Design review of the part built by this model. Coordinates are the model's own, in mm. Face numbers are marked on the shaded views. A direction names the side the tool comes from. Coordinates: 2 decimals unless noted, no trailing zeros. Loops run counter-clockwise (first coordinate to the right, second up) from the corner with the lowest first, then second, coordinate; pieces in that order, holes last. Notation, with made-up numbers: (-25, 4.25) -> (3, 4.25) arc R23 cw to (3, 20.25) -> close; hole circle Ø7 at (85, -11.5). An arc over 180 degrees is marked (long way). One line per item, written item: value. Start each with the question number.
1. Add section A-A on z = -70.5. Write out the cut boundary in (x, y).
2. Draft analysis for pull direction Y (two halves, no side actions). For the marked faces 1, 2, 3 and 4, state which applies: pulls with the +Y half, pulls with the -Y half, needs draft (parallel to the pull), parting line crosses it, or undercut.
3. Insertion check: pin 1 (6 mm diameter, centred on x = -157, z = -24, fed in from -Y); pin 2 (4 mm diameter, centred on y = -91.5, z = 2, fed in from +X); pin 3 (8 mm diameter, centred on x = -125, y = 0, fed in from +Z). Each pin has a flat end and moves straight along its axis. Give the tip position at first contact, or say it passes through.
4. Machinability: for the marked faces 5, 6, 7, 8 and 9, which of the approach directions +Z, -Z, +X, -X, +Y, -Y give a long, thin tool a straight path to every point of the face, cutting with its end or side? Answer none if there is none.
5. Add section B-B on z = 41. Write out the cut boundary in (x, y).
6. For probe 1 along Z at (x, y) = (-264.5, 45); probe 2 along X at (y, z) = (-70, -5.5); probe 3 along Y at (x, z) = (-195.5, 32), list the stretches that pass through material, from the lowest coordinate up.
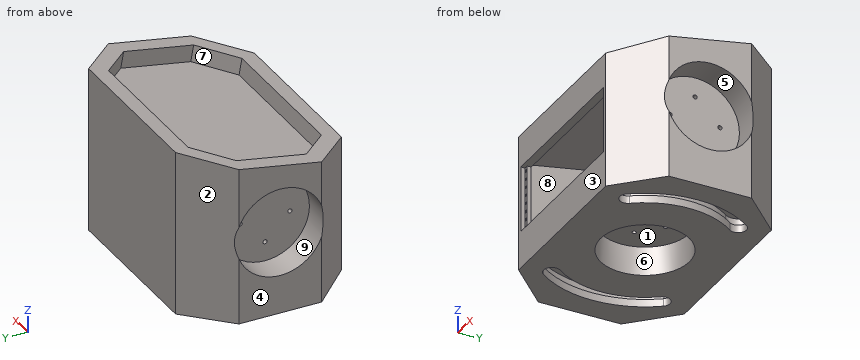
```python
from build123d import *

# Parameters (mm, degrees)
SKETCH1_W           = 200
SKETCH1_H           = 200
BOSS_EXTRUDE1_DEPTH = 150
SKETCH2_R           = 53.5
CUT_EXTRUDE1_DEPTH  = 35
CUT_EXTRUDE3_DEPTH  = 332.662479036
CHAMFER2_SIZE       = 50
CUT_EXTRUDE5_DEPTH  = 20
CUT_EXTRUDE6_DEPTH  = 20
BOSS_EXTRUDE3_DEPTH = 9.2
SKETCH11_R          = 53.5
CUT_EXTRUDE7_DEPTH  = 35
SKETCH12_R          = 2.5
CUT_EXTRUDE8_DEPTH  = 10
SKETCH13_R          = 2.5
CUT_EXTRUDE9_DEPTH  = 10
CUT_EXTRUDE10_DEPTH = 105
SKETCH15_W          = 180
SKETCH15_H          = 80
CUT_EXTRUDE11_DEPTH = 10
SKETCH17_W          = 5
SKETCH17_H          = 80
CUT_EXTRUDE12_DEPTH = 5
SKETCH17_3_R        = 1.5
CUT_EXTRUDE13_DEPTH = 10


with BuildPart() as part:
    # Sketch1 → Boss-Extrude1 (new body)
    with BuildSketch(Plane(origin=(0, 0, 0), x_dir=(0, 0, -1), z_dir=(1, 0, 0))):
        Rectangle(SKETCH1_W, SKETCH1_H)
    extrude(amount=-BOSS_EXTRUDE1_DEPTH)

    # Sketch2 → Cut-Extrude1 (cut)
    with BuildSketch(Plane(origin=(0, 0, 0), x_dir=(0, 0, -1), z_dir=(1, 0, 0))):
        Circle(SKETCH2_R)
    extrude(amount=-CUT_EXTRUDE1_DEPTH, mode=Mode.SUBTRACT)

    # Mirror1: part across plane


with BuildPart() as part_1:
    add(part.part)
    add(part.part.mirror(Plane(origin=(-150, 0, 0), x_dir=(0, 0, 1), z_dir=(1, 0, 0))))

    # Sketch6 → Cut-Extrude3 (cut, through all)
    with BuildSketch(Plane(origin=(0, 0, 0), x_dir=(0, 0, -1), z_dir=(1, 0, 0))):
        Polygon((-100, 100), (-64.734603858, -100), (-100, -100), align=None)
    extrude(amount=-CUT_EXTRUDE3_DEPTH, mode=Mode.SUBTRACT)

    # Chamfer2
    # the kernel refuses this chamfer: 50 mm, written as the material it takes off along each edge
    with BuildSketch(Plane(origin=(-300, 100, -228.584149398), x_dir=(-0.027495876610586594, -0.9996219169112966, 0), z_dir=(0, 0, 1))) as chamfer2_piece_1:
        Polygon((CHAMFER2_SIZE * 0.999621916911, CHAMFER2_SIZE * 0.0274958766106), (-CHAMFER2_SIZE * 0.0274958766106, CHAMFER2_SIZE * 0.999621916911), (0, 0), align=None)
    extrude(amount=457.168298797, mode=Mode.SUBTRACT)
    with BuildSketch(Plane(origin=(-300, -100, 193.318753257), x_dir=(0.9996219169112966, -0.02749587661058631, 0), z_dir=(0, 0, -1))) as chamfer2_piece_2:
        Polygon((CHAMFER2_SIZE * 0.999621916911, -CHAMFER2_SIZE * 0.0274958766106), (-CHAMFER2_SIZE * 0.0274958766106, -CHAMFER2_SIZE * 0.999621916911), (0, 0), align=None)
    extrude(amount=421.902902655, mode=Mode.SUBTRACT)
    with BuildSketch(Plane(origin=(0, -100, 193.318753257), x_dir=(-0.9996219169112966, -0.027495876610586317, 0), z_dir=(0, 0, -1))) as chamfer2_piece_3:
        Polygon((CHAMFER2_SIZE * 0.999621916911, CHAMFER2_SIZE * 0.0274958766106), (-CHAMFER2_SIZE * 0.0274958766106, CHAMFER2_SIZE * 0.999621916911), (0, 0), align=None)
    extrude(amount=421.902902655, mode=Mode.SUBTRACT)
    with BuildSketch(Plane(origin=(0, 100, -228.584149398), x_dir=(0.02749587661058637, -0.9996219169112966, 0), z_dir=(0, 0, 1))) as chamfer2_piece_4:
        Polygon((CHAMFER2_SIZE * 0.999621916911, -CHAMFER2_SIZE * 0.0274958766106), (-CHAMFER2_SIZE * 0.0274958766106, -CHAMFER2_SIZE * 0.999621916911), (0, 0), align=None)
    extrude(amount=457.168298797, mode=Mode.SUBTRACT)

    # Sketch8 → Cut-Extrude5 (cut)
    with BuildSketch(Plane(origin=(0, -14.085638206, 79.883623873), x_dir=(1, 0, 0), z_dir=(0, -0.17364817766693483, 0.9848077530122074))):
        Polygon((-280, -28.273659533), (-241.625912379, -67.239729309), (-58.966069777, -67.239729309), (-20, -28.865641689), (-20, 56.879523291), (-58.374087621, 95.845593068), (-241.033930223, 95.845593068), (-280, 57.471505447), align=None)
    extrude(amount=-CUT_EXTRUDE5_DEPTH, mode=Mode.SUBTRACT)

    # Sketch9 → Cut-Extrude6 (cut)
    with BuildSketch(Plane(origin=(0, 0, -100), x_dir=(-1, 0, 0), z_dir=(0, 0, -1))):
        with BuildLine():
            ThreePointArc((249.615655403, -75.509742408), (275, 0), (249.615655403, 75.509742408))
            ThreePointArc((249.615655403, 75.509742408), (228.600607666, 78.402451968), (225.707898107, 57.38740423))
            ThreePointArc((225.707898107, 57.38740423), (245, 0), (225.707898107, -57.38740423))
            ThreePointArc((225.707898107, -57.38740423), (228.600607666, -78.402451968), (249.615655403, -75.509742408))
        make_face()
        with BuildLine():
            ThreePointArc((50.384344597, 75.509742408), (71.399392334, 78.402451968), (74.292101893, 57.38740423))
            ThreePointArc((74.292101893, 57.38740423), (55, 0), (74.292101893, -57.38740423))
            ThreePointArc((74.292101893, -57.38740423), (71.399392334, -78.402451968), (50.384344597, -75.509742408))
            ThreePointArc((50.384344597, -75.509742408), (25, 0), (50.384344597, 75.509742408))
        make_face()
    extrude(amount=-CUT_EXTRUDE6_DEPTH, mode=Mode.SUBTRACT)

    # Sketch10 → Boss-Extrude3 (add)
    # profile 1 of 2: a face of its own
    with BuildSketch(Plane(origin=(0, 0, -100), x_dir=(-1, 0, 0), z_dir=(0, 0, -1))):
        with BuildLine():
            ThreePointArc((74.292101893, 57.38740423), (55, 0), (74.292101893, -57.38740423))
            ThreePointArc((74.292101893, -57.38740423), (71.399392334, -78.402451968), (50.384344597, -75.509742408))
            ThreePointArc((50.384344597, -75.509742408), (25, 0), (50.384344597, 75.509742408))
            ThreePointArc((50.384344597, 75.509742408), (71.399392334, 78.402451968), (74.292101893, 57.38740423))
        make_face()
        with BuildLine():
            ThreePointArc((70.307475677, 60.407793927), (50, 0), (70.307475677, -60.407793927))
            ThreePointArc((70.307475677, -60.407793927), (68.379002638, -74.417825752), (54.368970813, -72.489352712))
            ThreePointArc((54.368970813, -72.489352712), (30, 0), (54.368970813, 72.489352712))
            ThreePointArc((54.368970813, 72.489352712), (68.379002638, 74.417825752), (70.307475677, 60.407793927))
        make_face(mode=Mode.SUBTRACT)
    # profile 2 of 2: a face of its own
    with BuildSketch(Plane(origin=(0, 0, -100), x_dir=(-1, 0, 0), z_dir=(0, 0, -1))):
        with BuildLine():
            ThreePointArc((249.615655403, 75.509742408), (228.600607666, 78.402451968), (225.707898107, 57.38740423))
            ThreePointArc((225.707898107, 57.38740423), (245, 0), (225.707898107, -57.38740423))
            ThreePointArc((225.707898107, -57.38740423), (228.600607666, -78.402451968), (249.615655403, -75.509742408))
            ThreePointArc((249.615655403, -75.509742408), (275, 0), (249.615655403, 75.509742408))
        make_face()
        with BuildLine():
            ThreePointArc((245.631029187, 72.489352712), (231.620997362, 74.417825752), (229.692524323, 60.407793927))
            ThreePointArc((229.692524323, 60.407793927), (250, 0), (229.692524323, -60.407793927))
            ThreePointArc((229.692524323, -60.407793927), (231.620997362, -74.417825752), (245.631029187, -72.489352712))
            ThreePointArc((245.631029187, -72.489352712), (270, 0), (245.631029187, 72.489352712))
        make_face(mode=Mode.SUBTRACT)
    extrude(amount=-BOSS_EXTRUDE3_DEPTH)

    # Sketch11 → Cut-Extrude7 (cut)
    with BuildSketch(Plane(origin=(0, 0, -100), x_dir=(-1, 0, 0), z_dir=(0, 0, -1))):
        with Locations((150, 0)):
            Circle(SKETCH11_R)
    extrude(amount=-CUT_EXTRUDE7_DEPTH, mode=Mode.SUBTRACT)

    # Sketch12 → Cut-Extrude8 (cut)
    with BuildSketch(Plane(origin=(-35, 0, 0), x_dir=(0, 0, -1), z_dir=(1, 0, 0))):
        with Locations((0, 30)):
            Circle(SKETCH12_R)
        with Locations((30, 0)):
            Circle(SKETCH12_R)
        with Locations((0, -30)):
            Circle(SKETCH12_R)
        with Locations((-30, 0)):
            Circle(SKETCH12_R)
    cut_extrude8 = extrude(amount=-CUT_EXTRUDE8_DEPTH, mode=Mode.SUBTRACT)

    # Mirror2: Cut-Extrude8 across plane
    add(cut_extrude8.mirror(Plane(origin=(-150, 0, 0), x_dir=(0, 0, 1), z_dir=(1, 0, 0))), mode=Mode.SUBTRACT)

    # Sketch13 → Cut-Extrude9 (cut)
    with BuildSketch(Plane(origin=(0, 0, -65), x_dir=(-1, 0, 0), z_dir=(0, 0, -1))):
        with Locations((150, 25)):
            Circle(SKETCH13_R)
        with Locations((150, -25)):
            Circle(SKETCH13_R)
        with Locations((175, 0)):
            Circle(SKETCH13_R)
        with Locations((125, 0)):
            Circle(SKETCH13_R)
    extrude(amount=-CUT_EXTRUDE9_DEPTH, mode=Mode.SUBTRACT)

    # Sketch14 → Cut-Extrude10 (cut, symmetric)
    with BuildSketch(Plane(origin=(-150, 0, 0), x_dir=(0, 0, -1), z_dir=(1, 0, 0))):
        Polygon((-67.773931836, 90), (-36.035075309, -90), (55, -90), (55, 90), align=None)
    extrude(amount=CUT_EXTRUDE10_DEPTH, both=True, mode=Mode.SUBTRACT)

    # Sketch15 → Cut-Extrude11 (cut)
    with BuildSketch(Plane.XZ.offset(100)):
        with Locations((-150, -15)):
            Rectangle(SKETCH15_W, SKETCH15_H)
    extrude(amount=-CUT_EXTRUDE11_DEPTH, mode=Mode.SUBTRACT)

    # Sketch17 → Cut-Extrude12 (cut)
    with BuildSketch(Plane.XZ.offset(100)):
        with Locations((-242.5, -15)):
            Rectangle(SKETCH17_W, SKETCH17_H)
        with Locations((-57.5, -15)):
            Rectangle(SKETCH17_W, SKETCH17_H)
    extrude(amount=-CUT_EXTRUDE12_DEPTH, mode=Mode.SUBTRACT)

    # Sketch17<3> → Cut-Extrude13 (cut)
    with BuildSketch(Plane.XZ.offset(100)):
        with Locations(Location((-57.5, -10, 0), (0, 0, 270))):
            Circle(SKETCH17_3_R)
        with Locations(Location((-242.5, 20, 0), (0, 0, 270))):
            Circle(SKETCH17_3_R)
        with Locations(Location((-242.5, 10, 0), (0, 0, 270))):
            Circle(SKETCH17_3_R)
        with Locations(Location((-242.5, 0, 0), (0, 0, 270))):
            Circle(SKETCH17_3_R)
        with Locations(Location((-242.5, -10, 0), (0, 0, 270))):
            Circle(SKETCH17_3_R)
        with Locations(Location((-242.5, -20, 0), (0, 0, 270))):
            Circle(SKETCH17_3_R)
        with Locations(Location((-242.5, -30, 0), (0, 0, 270))):
            Circle(SKETCH17_3_R)
        with Locations(Location((-242.5, -40, 0), (0, 0, 270))):
            Circle(SKETCH17_3_R)
        with Locations(Location((-242.5, -50, 0), (0, 0, 270))):
            Circle(SKETCH17_3_R)
        with Locations(Location((-57.5, -50, 0), (0, 0, 270))):
            Circle(SKETCH17_3_R)
        with Locations(Location((-57.5, -40, 0), (0, 0, 270))):
            Circle(SKETCH17_3_R)
        with Locations(Location((-57.5, -30, 0), (0, 0, 270))):
            Circle(SKETCH17_3_R)
        with Locations(Location((-57.5, -20, 0), (0, 0, 270))):
            Circle(SKETCH17_3_R)
        with Locations(Location((-57.5, 0, 0), (0, 0, 270))):
            Circle(SKETCH17_3_R)
        with Locations(Location((-57.5, 10, 0), (0, 0, 270))):
            Circle(SKETCH17_3_R)
        with Locations(Location((-57.5, 20, 0), (0, 0, 270))):
            Circle(SKETCH17_3_R)
    extrude(amount=-CUT_EXTRUDE13_DEPTH, mode=Mode.SUBTRACT)


solid = part_1.part
```
Worked answers:
1. outline: (-300, -50) -> (-250, -100) -> (-50, -100) -> (0, -50) -> (0, 50) -> (-50, 100) -> (-250, 100) -> (-300, 50) -> close; hole circle Ø107 at (-150, 0)
2. face 1: undercut
2. face 2: pulls with the +Y half
2. face 3: pulls with the -Y half
2. face 4: needs draft
3. pin 1: stops at y = 90
3. pin 2: stops at x = -39.5
3. pin 3: stops at z = 62.76
4. face 5: +X
4. face 6: -Z
4. face 7: +Z
4. face 8: none
4. face 9: -X
5. outline: (-300, -50) -> (-250, -100) -> (-50, -100) -> (0, -50) -> (0, -34.37) -> (-35, -34.37) -> (-35, 34.37) -> (0, 34.37) -> (0, 50) -> (-50, 100) -> (-250, 100) -> (-300, 50) -> (-300, 34.37) -> (-265, 34.37) -> (-265, -34.37) -> (-300, -34.37) -> close; hole (-255, -61.84) -> (-45, -61.84) -> (-45, 90) -> (-255, 90) -> close
6. probe 1: z = -100 to -90.8, -80 to 69.99
6. probe 2: x = -280 to -255, -45 to -20
6. probe 3: y = -100 to -90, 90 to 100
